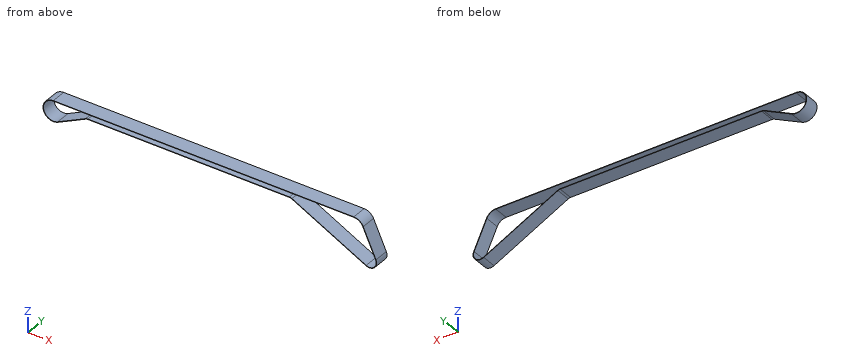
```python
from build123d import *

# Parameters (mm, degrees)
BOSS_EXTRUDE1_DEPTH = 15


with BuildPart() as part:
    # Sketch1 → Boss-Extrude1 (new body)
    with BuildSketch(Plane(origin=(0, 0, 0), x_dir=(1, 0, 0), z_dir=(0, 1, 0))):
        with BuildLine():
            Line((238.84, -5), (35, -5))
            ThreePointArc((35, -5), (33.863075353, -4.869024784), (32.785714286, -4.482960938))
            Line((32.785714286, -4.482960938), (4.65, 9.414217971))
            ThreePointArc((4.65, 9.414217971), (-10.224952046, 2.38754176), (0, -10.5))
            Line((0, -10.5), (303.94, -10.5))
            ThreePointArc((303.94, -10.5), (309.61007222, -8.837436338), (313.484552814, -4.376244004))
            Line((313.484552814, -4.376244004), (326.437537724, 23.874111425))
            ThreePointArc((326.437537724, 23.874111425), (324.816305533, 32.408179805), (316.224290262, 33.687238247))
            Line((316.224290262, 33.687238247), (241.103806492, -4.458158831))
            ThreePointArc((241.103806492, -4.458158831), (240.0038741, -4.862653296), (238.84, -5))
        make_face()
        with BuildLine():
            Line((0, -10), (303.94, -10))
            ThreePointArc((303.94, -10), (309.340068781, -8.416606036), (313.030050299, -4.167851433))
            Line((313.030050299, -4.167851433), (325.983035209, 24.082503997))
            ThreePointArc((325.983035209, 24.082503997), (324.469885164, 32.047634485), (316.450670911, 33.241422364))
            Line((316.450670911, 33.241422364), (241.330187142, -4.903974714))
            ThreePointArc((241.330187142, -4.903974714), (240.12026151, -5.348918626), (238.84, -5.5))
            Line((238.84, -5.5), (35, -5.5))
            ThreePointArc((35, -5.5), (33.749382888, -5.355927262), (32.564285714, -4.931257032))
            Line((32.564285714, -4.931257032), (4.428571429, 8.965921877))
            ThreePointArc((4.428571429, 8.965921877), (-9.738049568, 2.273849295), (0, -10))
        make_face(mode=Mode.SUBTRACT)
    extrude(amount=BOSS_EXTRUDE1_DEPTH)


solid = part.part
```
Geometry: final body of the model. Coordinates: model frame, mm. Round coordinates to 2 decimals unless told otherwise and drop trailing zeros. Write each loop counter-clockwise with the first axis right and the second up, starting at its lowest first coordinate (ties: lowest second). Pieces come first, ordered by that corner, then holes.
Item 1: Pin query (flat end, axial travel): P1, Ø1, axis at y = 9.5, z = -14, coming from the -X side; P2, Ø2, axis at x = 87.5, y = 13, coming from the -Z side; P3, Ø2, axis at x = 279.5, y = 5, coming from the -Z side; P4, Ø12, axis at x = 0, z = 0, coming from the +Y side. Return the tip coordinate at first contact, or that it passes through.
Item 2: Section query A-A (x = 84.5). Return loops of the section in (y, z).
Item 3: Section query C-C (y = 3.5). Return loops of the section in (x, z), plus the area to 3 significant figures.
Item 4: Material intervals for L1, parallel to Z at x = 48, y = 1; L2, parallel to Z at x = 0, y = 3; L3, parallel to X at y = 8.5, z = 0, sorted ascending.
Item 5: Section query B-B (z = 0). Return loops of the section in (x, y).
Item 6: Section query D-D (z = -18.5). Return loops of the section in (x, y).
Completed:
1. P1: stops at x = 276.47
1. P2: stops at z = 5
1. P3: stops at z = -15.55
1. P4: passes through
2. outline: (0, 5) - (15, 5) - (15, 5.5) - (0, 5.5) - close; (0, 10) - (15, 10) - (15, 10.5) - (0, 10.5) - close
3. outline: (0, 10.5) arc R10.5 ccw (long way) to (4.65, -9.41) - (32.79, 4.48) arc R5 cw to (35, 5) - (238.84, 5) arc R5 cw to (241.1, 4.46) - (316.22, -33.69) arc R7.5 ccw to (326.44, -23.87) - (313.48, 4.38) arc R10.5 ccw to (303.94, 10.5) - close; hole (0, 10) arc R10 ccw (long way) to (4.43, -8.97) - (32.56, 4.93) arc R5.5 cw to (35, 5.5) - (238.84, 5.5) arc R5.5 cw to (241.33, 4.9) - (316.45, -33.24) arc R7 ccw to (325.98, -24.08) - (313.03, 4.17) arc R10 ccw to (303.94, 10) - close
3. area: 363 mm2
4. L1: z = 5 to 5.5, 10 to 10.5
4. L2: z = -10.5 to -10, 10 to 10.5
4. L3: x = -10.5 to -10, 22.58 to 23.71, 249.88 to 250.99, 314.94 to 315.49
5. outline: (-10.5, 0) - (-10, 0) - (-10, 15) - (-10.5, 15) - close; (22.58, 0) - (23.71, 0) - (23.71, 15) - (22.58, 15) - close; (249.88, 0) - (250.99, 0) - (250.99, 15) - (249.88, 15) - close; (314.94, 0) - (315.49, 0) - (315.49, 15) - (314.94, 15) - close
6. outline: (286.32, 0) - (287.42, 0) - (287.42, 15) - (286.32, 15) - close; (323.42, 0) - (323.97, 0) - (323.97, 15) - (323.42, 15) - close
